Check sheet for the modelled part. Datum: model origin and axes. Units: mm. A direction names the side the tool comes from. Round coordinates to 2 decimals unless told otherwise and drop trailing zeros. Write each loop counter-clockwise with the first axis right and the second up, starting at its lowest first coordinate (ties: lowest second). Pieces come first, ordered by that corner, then holes. Notation, with made-up numbers: M 36.5,28 L 85.5,28 A7 ccw 85.5,34 Z; hole C -25,13 d7. An arc over 180 degrees is marked long. Answer in a Markdown table with one row per item.
```python
from build123d import *

# Parameters (mm, degrees)
F1_DEPTH       = 7.3
F1_DEPTH_BACK  = 7.3
F3_DEPTH       = 6
F3_DEPTH_BACK  = 6
F5_DEPTH       = 10
F5_DEPTH_BACK  = 10
F8_DEPTH       = 25
F9_R           = 2.5
F10_DEPTH      = 2.5
F10_DEPTH_BACK = 2.5
F11_T1_DEPTH   = 6.5
F11_T6_DEPTH   = 12.7132034356
F11_S7_R       = 5
F11_T8_DEPTH   = 8
F11_S10_R      = 17
F11_T11_DEPTH  = 8
F11_T15_DEPTH  = 8.5710678119
F11_T20_DEPTH  = 12.7132034356
F11_S21_R      = 5
F11_T22_DEPTH  = 8
F11_S24_R      = 17
F11_T25_DEPTH  = 8
F11_T29_DEPTH  = 8.5710678119
F11_T31_DEPTH  = 10.6421356237
F12_R          = 1
F13_R          = 2
F14_DEPTH      = 5
F15_R          = 1.05
F16_DEPTH      = 3
F16_DEPTH_BACK = 10
F17_SIZE       = 1
F19_START      = 3.8
F18_R          = 3
F19_DEPTH      = 4
F21_START      = 4.5
F21_DEPTH      = 2.6
F22_R          = 1.29999


# Not quite as in the source:
# - a fillet or chamfer that OpenCascade refuses, or shapes differently, is made with other operations: its cross-section is extruded or revolved along the edge and cut away or added
# - a fillet or chamfer is up to 0.001 mm smaller than in the source, because OpenCascade refuses the exact size


with BuildPart() as f1:
    # F0 (on Front) → F1 (new body, two sides)
    with BuildSketch(Plane.XZ) as f1_sk:
        with BuildLine():
            Line((-7.2480415045, 9.479816391), (-6, 0))
            Line((-6, 0), (6, 0))
            Line((6, 0), (9.6197658273, 19.3731186918))
            ThreePointArc((9.6197658273, 19.3731186918), (9.492555749, 19.6769779623), (9.1631662961, 19.6809084286))
            ThreePointArc((9.1631662961, 19.6809084286), (-0.3536100614, 17.0036780472), (-9.750799418, 20.0744152471))
            Line((-9.750799418, 20.0744152471), (-25.666835692, 22.7954629152))
            ThreePointArc((-25.666835692, 22.7954629152), (-26.3420622378, 23.0419468668), (-26.8865335991, 23.511240126))
            ThreePointArc((-26.8865335991, 23.511240126), (-33.4498266444, 23.0245236782), (-30.6740705867, 17.0572054525))
            Line((-30.6740705867, 17.0572054525), (-11.362677578, 13.7556786143))
            ThreePointArc((-11.362677578, 13.7556786143), (-8.6024605414, 12.2941429125), (-7.2480415045, 9.479816391))
        make_face()
    extrude(amount=F1_DEPTH)
    extrude(f1_sk.sketch, amount=-F1_DEPTH_BACK)

    # F2 (on Front) → F3 (cut, two sides)
    with BuildSketch(Plane.XZ) as f3_sk:
        Polygon((15, 1.3), (15, 78.0352148958), (0, 78.0352148958), (-11, 13.6936742961), (-11, 1.3), align=None)
    extrude(amount=F3_DEPTH, mode=Mode.SUBTRACT)
    extrude(f3_sk.sketch, amount=-F3_DEPTH_BACK, mode=Mode.SUBTRACT)

    # F4 (on Front) → F5 (cut, two sides)
    with BuildSketch(Plane.XZ) as f5_sk:
        with BuildLine():
            Line((0, 18), (-1.125, 18))
            Line((-1.125, 18), (-1.125, 15.2))
            ThreePointArc((-1.125, 15.2), (-1.0664213562, 15.0585786438), (-0.925, 15))
            Line((-0.925, 15), (0, 15))
            Line((0, 15), (0.925, 15))
            ThreePointArc((0.925, 15), (1.0664213562, 15.0585786438), (1.125, 15.2))
            Line((1.125, 15.2), (1.125, 18))
            Line((1.125, 18), (0, 18))
        make_face()
        with BuildLine():
            ThreePointArc((0, 11.5), (-1.50260191, 10.87760191), (-2.125, 9.375))
            Line((-2.125, 9.375), (-2.125, 5.125))
            ThreePointArc((-2.125, 5.125), (-1.50260191, 3.62239809), (0, 3))
            ThreePointArc((0, 3), (1.50260191, 3.62239809), (2.125, 5.125))
            Line((2.125, 5.125), (2.125, 9.375))
            ThreePointArc((2.125, 9.375), (1.50260191, 10.87760191), (0, 11.5))
        make_face()
    extrude(amount=F5_DEPTH, mode=Mode.SUBTRACT)
    extrude(f5_sk.sketch, amount=-F5_DEPTH_BACK, mode=Mode.SUBTRACT)

    # F7 (on offset) → F8 (cut)
    with BuildSketch(Plane(origin=(1.9622434031, 0, 11.4776148716), x_dir=(0.9856986369, 0, -0.1685176467), z_dir=(-0.1685176467, 0, -0.9856986369))):
        Polygon((-41.9907133171, -7.3), (-13.6887884036, -7.3), (-17.1887884036, -3.8), (-41.9907133171, -3.8), align=None)
        Polygon((-41.9907133171, 7.3), (-41.9907133171, 3.8), (-17.1887884036, 3.8), (-13.6887884036, 7.3), align=None)
        Polygon((-16.6503107725, -2.5), (-13.1503107725, -6), (-13.1503107725, 0), (-13.1503107725, 6), (-16.6503107725, 2.5), (-41.9907133171, 2.5), (-41.9907133171, 0), (-41.9907133171, -2.5), align=None)
    extrude(amount=-F8_DEPTH, mode=Mode.SUBTRACT)

    # F9 (on Front) → F10 (join, two sides)
    with BuildSketch(Plane.XZ) as f10_sk:
        with Locations((-30, 21)):
            Circle(F9_R)
    extrude(amount=F10_DEPTH)
    extrude(f10_sk.sketch, amount=-F10_DEPTH_BACK)

    # F11: fillet of radius 2 on 8 edges, made by hand

    # F11_s2 → F11_t1 (join)
    with BuildSketch(Plane(origin=(1.9622434031, 0, 11.4776148716), x_dir=(0, 1, 0), z_dir=(0.1685176467, 0, 0.9856986369))):
        with BuildLine():
            ThreePointArc((3.8, 18.0172155284), (3.952240935, 17.2518486636), (4.3857864376, 16.603001966))
            Line((4.3857864376, 16.603001966), (3.8, 17.1887884036))
            Line((3.8, 17.1887884036), (3.8, 18.0172155284))
        make_face()
        with BuildLine():
            ThreePointArc((-4.3857864376, 16.603001966), (-3.952240935, 17.2518486636), (-3.8, 18.0172155284))
            Line((-3.8, 18.0172155284), (-3.8, 17.1887884036))
            Line((-3.8, 17.1887884036), (-4.3857864376, 16.603001966))
        make_face()
    extrude(amount=F11_T1_DEPTH)


with BuildPart() as f11_tool4:
    # F11_s5 → F11_t6 (new body)
    with BuildSketch(Plane(origin=(3.0576081065, 0, 17.8846560114), x_dir=(0, 1, 0), z_dir=(-0.1685176467, 0, -0.9856986369))):
        with BuildLine():
            ThreePointArc((-6, -12.3218836478), (-5.847759065, -13.0872505125), (-5.4142135624, -13.7360972102))
            Line((-5.4142135624, -13.7360972102), (-6, -13.1503107725))
            Line((-6, -13.1503107725), (-6, -12.3218836478))
        make_face()
    extrude(amount=F11_T6_DEPTH)

    # F11_s7 → F11_t8 (cut, symmetric)
    with BuildSketch(Plane.XZ.offset(5.7)):
        with Locations((-12.2052658114, 8.8271854299)):
            Circle(F11_S7_R)
    extrude(amount=F11_T8_DEPTH, both=True, mode=Mode.SUBTRACT)

    split(bisect_by=Plane.YZ.offset(-11), keep=Keep.TOP)

    # F11_s10 → F11_t11 (cut, symmetric)
    with BuildSketch(Plane.XZ.offset(5.7)):
        with Locations((0, 34)):
            Circle(F11_S10_R)
    extrude(amount=F11_T11_DEPTH, both=True, mode=Mode.SUBTRACT)


with BuildPart() as f1_1:
    add(f1.part)

    # F11_t3: union F11_tool4
    add(f11_tool4.part)


with BuildPart() as f11_tool13:
    # F11_s14 → F11_t15 (new body)
    with BuildSketch(Plane(origin=(3.4066195803, 0, 19.9261047304), x_dir=(0, 1, 0), z_dir=(-0.1685176467, 0, -0.9856986369))):
        with BuildLine():
            ThreePointArc((-6, -12.3218836478), (-5.847759065, -13.0872505125), (-5.4142135624, -13.7360972102))
            Line((-5.4142135624, -13.7360972102), (-6, -13.1503107725))
            Line((-6, -13.1503107725), (-6, -12.3218836478))
        make_face()
    extrude(amount=F11_T15_DEPTH)

    split(bisect_by=Plane.YZ.offset(-11), keep=Keep.BOTTOM)


with BuildPart() as f1_2:
    add(f1_1.part)

    # F11_t12: union F11_tool13
    add(f11_tool13.part)


with BuildPart() as f11_tool18:
    # F11_s19 → F11_t20 (new body)
    with BuildSketch(Plane(origin=(3.0576081065, 0, 17.8846560114), x_dir=(0, 1, 0), z_dir=(-0.1685176467, 0, -0.9856986369))):
        with BuildLine():
            ThreePointArc((6, -12.3218836478), (5.847759065, -13.0872505125), (5.4142135624, -13.7360972102))
            Line((5.4142135624, -13.7360972102), (6, -13.1503107725))
            Line((6, -13.1503107725), (6, -12.3218836478))
        make_face()
    extrude(amount=F11_T20_DEPTH)

    # F11_s21 → F11_t22 (cut, symmetric)
    with BuildSketch(Plane.XZ.offset(-5.7)):
        with Locations((-12.2052658114, 8.8271854299)):
            Circle(F11_S21_R)
    extrude(amount=F11_T22_DEPTH, both=True, mode=Mode.SUBTRACT)

    split(bisect_by=Plane.YZ.offset(-11), keep=Keep.TOP)

    # F11_s24 → F11_t25 (cut, symmetric)
    with BuildSketch(Plane.XZ.offset(-5.7)):
        with Locations((0, 34)):
            Circle(F11_S24_R)
    extrude(amount=F11_T25_DEPTH, both=True, mode=Mode.SUBTRACT)


with BuildPart() as f1_3:
    add(f1_2.part)

    # F11_t17: union F11_tool18
    add(f11_tool18.part)


with BuildPart() as f11_tool27:
    # F11_s28 → F11_t29 (new body)
    with BuildSketch(Plane(origin=(3.4066195803, 0, 19.9261047304), x_dir=(0, 1, 0), z_dir=(-0.1685176467, 0, -0.9856986369))):
        with BuildLine():
            ThreePointArc((6, -12.3218836478), (5.847759065, -13.0872505125), (5.4142135624, -13.7360972102))
            Line((5.4142135624, -13.7360972102), (6, -13.1503107725))
            Line((6, -13.1503107725), (6, -12.3218836478))
        make_face()
    extrude(amount=F11_T29_DEPTH)

    split(bisect_by=Plane.YZ.offset(-11), keep=Keep.BOTTOM)


with BuildPart() as f1_4:
    add(f1_3.part)

    # F11_t26: union F11_tool27
    add(f11_tool27.part)

    # F11_s32 → F11_t31 (cut)
    with BuildSketch(Plane(origin=(1.6132319293, 0, 9.4361661525), x_dir=(0, 1, 0), z_dir=(0.1685176467, 0, 0.9856986369))):
        with BuildLine():
            ThreePointArc((6.7142135624, 14.2745748413), (7.147759065, 13.6257281436), (7.3, 12.8603612789))
            Line((7.3, 12.8603612789), (7.3, 13.6887884036))
            Line((7.3, 13.6887884036), (6.7142135624, 14.2745748413))
        make_face()
        with BuildLine():
            ThreePointArc((-2.5, 17.4787378973), (-2.652240935, 16.7133710326), (-3.0857864376, 16.0645243349))
            Line((-3.0857864376, 16.0645243349), (-2.5, 16.6503107725))
            Line((-2.5, 16.6503107725), (-2.5, 17.4787378973))
        make_face()
        with BuildLine():
            ThreePointArc((-6.7142135624, 14.2745748413), (-7.147759065, 13.6257281436), (-7.3, 12.8603612789))
            Line((-7.3, 12.8603612789), (-7.3, 13.6887884036))
            Line((-7.3, 13.6887884036), (-6.7142135624, 14.2745748413))
        make_face()
        with BuildLine():
            ThreePointArc((2.5, 17.4787378973), (2.652240935, 16.7133710326), (3.0857864376, 16.0645243349))
            Line((3.0857864376, 16.0645243349), (2.5, 16.6503107725))
            Line((2.5, 16.6503107725), (2.5, 17.4787378973))
        make_face()
    extrude(amount=F11_T31_DEPTH, mode=Mode.SUBTRACT)

    # F12
    f12_edges = [f1_4.edges().sort_by_distance(p)[0] for p in [
        (0.035875, 6, 1.3),
        (0, -7.3, 0),
        (0.035875, -6, 1.3),
        (0, 7.3, 0),
    ]]
    fillet(f12_edges, radius=F12_R)

    # F13 (on Top) → F14 (cut)
    with BuildSketch(Plane.XY):
        Circle(F13_R)
    extrude(amount=F14_DEPTH, mode=Mode.SUBTRACT)

    # F15 (on Front) → F16 (cut, two sides)
    with BuildSketch(Plane.XZ) as f16_sk:
        with Locations((-30, 21)):
            Circle(F15_R)
    extrude(amount=F16_DEPTH, mode=Mode.SUBTRACT)
    extrude(f16_sk.sketch, amount=-F16_DEPTH_BACK, mode=Mode.SUBTRACT)

    # F17
    f17_edges = [f1_4.edges().sort_by_distance(p)[0] for p in [
        (-31.05, 3.8, 21),
    ]]
    chamfer(f17_edges, length=F17_SIZE)

    # F18 (on Front) → F19 (join)
    with BuildSketch(Plane.XZ.offset(F19_START)):
        with Locations((-30, 21)):
            Circle(F18_R)
    extrude(amount=F19_DEPTH)

    # F20 (on Front) → F21 (cut)
    with BuildSketch(Plane.XZ.offset(F21_START)):
        Polygon((-40.5470757535, 15.9000791133), (-31.814414217, 13.7227820529), (-28.185585783, 28.2772179471), (-36.9182473195, 30.4545150075), align=None)
    extrude(amount=F21_DEPTH, mode=Mode.SUBTRACT)

    # F22 (radius 1.3 in the source; OpenCascade refuses exactly that, so slightly less here)
    f22_edges = [f1_4.edges().sort_by_distance(p)[0] for p in [
        (-30, -4.5, 21),
        (-30, -7.1, 21),
    ]]
    fillet(f22_edges, radius=F22_R)


solid = f1_4.part
```
1. Section check B-B, the plane z = 8.75. Record the cut outline in (x, y) (3 decimals), and give its area (3 significant figures).
Found:
| item | result |
|---|---|
| outline | M -7.152,-7.3 L -2.125,-7.3 L -2.125,-6 L -7.152,-6 Z; M -7.152,6 L -2.125,6 L -2.125,7.3 L -7.152,7.3 Z; M 2.125,-7.3 L 7.635,-7.3 L 7.635,-6 L 2.125,-6 Z; M 2.125,6 L 7.635,6 L 7.635,7.3 L 2.125,7.3 Z |
| area | 27.4 mm2 |
2. Section check C-C, the plane x = -22. Record the cut outline in (y, z), and give its area (3 significant figures).
Found:
| item | result |
|---|---|
| outline | M -3.8,15.57 L -2.5,15.57 L -2.5,22.17 L -3.8,22.17 Z; M 2.5,15.57 L 3.8,15.57 L 3.8,22.17 L 2.5,22.17 Z |
| area | 17.1 mm2 |
3. Section check A-A, the plane y = -1.5. Count the separate pieces of the cut face and the enclosed holes in it, and give its area (3 significant figures).
Found:
| item | result |
|---|---|
| separate pieces | 4 |
| enclosed holes | 1 |
| area | 28.6 mm2 |
4. Go/stop test with flat-tipped pins: pin 1 (8 mm diameter, centred on x = -11, y = 1, fed in from -Z); pin 2 (8 mm diameter, centred on x = -1, y = 1, fed in from +Z); pin 3 (0.6 mm diameter, centred on y = -7, z = 15.5, fed in from +X). Record where each tip stops, or that it passes through.
Found:
| item | result |
|---|---|
| pin 1 | stops at z = 13.68 |
| pin 2 | stops at z = 1.3 |
| pin 3 | stops at x = 8.95 |
5. Draft check along Z on faces 5 (the face through (2.125, -7, 7)), 6 (the face through (0.114, 7.015, 0.301)), 7 (the face through (-1, 7.3, 13)), 8 (the face through (-30.35, -4.89, 21.13)). Enter one of: +Z half, -Z half, draft (parallel to the pull), parting line (faces both ways), or undercut.
Found:
| item | result |
|---|---|
| face 5 | undercut |
| face 6 | -Z half |
| face 7 | draft |
| face 8 | +Z half |
6. Access from +Z, -Z, +X, -X, +Y, -Y to the whole of each face (thin tool, end or side, straight path). Record for faces 1 (the face through (0.153, -5.699, 1.585)), 2 (the face through (-27.23, -5.77, 19.85)), 3 (the face through (-13.98, 2.65, 17.45)), 4 (the face through (-1.125, -7, 16)).
Found:
| item | result |
|---|---|
| face 1 | +Z, +X, -X |
| face 2 | -Y |
| face 3 | -Z, +X |
| face 4 | +Z, +Y, -Y |
7. Scan lines: L1, parallel to Z at x = -30, y = 0.65; L2, parallel to Y at x = -22, z = 18.25; L3, parallel to Y at x = -10.5, z = 15.5. Record each from-to range of solid material in increasing order.
Found:
| item | result |
|---|---|
| L1 | z = 18.5 to 19.95, 22.05 to 23.5 |
| L2 | y = -3.8 to -2.5, 2.5 to 3.8 |
| L3 | y = -7.3 to -5.89, 5.89 to 7.3 |
